from build123d import *

# Parameters (mm, degrees)
SKETCH2_R             = 25.4
BOSS_EXTRUDE2_DEPTH   = 6
SKETCH3_R             = 15
BOSS_EXTRUDE3_DEPTH   = 60.5
SKETCH4_R             = 10.315
CUT_EXTRUDE1_DEPTH    = 38.1
SKETCH5_R             = 7.07
CUT_EXTRUDE2_DEPTH    = 53.363441445
F_4_0MM_DOWEL_HOLE1_D = 4
CIRPATTERN1_COUNT     = 8
CIRPATTERN2_COUNT     = 6
CUT_EXTRUDE3_REACH    = 72.36


with BuildPart() as part:
    # Sketch2 → Boss-Extrude2 (new body)
    with BuildSketch(Plane(origin=(0, 0, 0), x_dir=(1, 0, 0), z_dir=(0, 1, 0))):
        with Locations(Location((0, 0, 0), (0, 0, 270))):
            Circle(SKETCH2_R)
    extrude(amount=BOSS_EXTRUDE2_DEPTH)

    # Sketch3 → Boss-Extrude3 (add)
    with BuildSketch(Plane.XZ):
        with Locations(Location((0, 0, 0), (0, 0, 270))):
            Circle(SKETCH3_R)
    extrude(amount=-BOSS_EXTRUDE3_DEPTH)

    # Sketch4 → Cut-Extrude1 (cut)
    with BuildSketch(Plane.XZ):
        with Locations(Location((0, 0, 0), (0, 0, 270))):
            Circle(SKETCH4_R)
    extrude(amount=-CUT_EXTRUDE1_DEPTH, mode=Mode.SUBTRACT)

    # Sketch5 → Cut-Extrude2 (cut, through all)
    with BuildSketch(Plane.XZ.offset(-38.1)):
        with Locations(Location((0, 0, 0), (0, 0, 270))):
            Circle(SKETCH5_R)
    extrude(amount=-CUT_EXTRUDE2_DEPTH, mode=Mode.SUBTRACT)

    # Ø4.0mm Dowel Hole1 (through all)
    with Locations(Plane(origin=(0, 0, 0), x_dir=(-1, 0, 0), z_dir=(0, -1, 0))):
        with Locations((0, 20.7)):
            f_4_0mm_dowel_hole1 = Hole(F_4_0MM_DOWEL_HOLE1_D / 2)

    # CirPattern1: Ø4.0mm Dowel Hole1 ×8 about axis
    cirpattern1_axis = Axis((0, 0, 0), (0, 1, 0))
    for i in range(1, CIRPATTERN1_COUNT):
        add(f_4_0mm_dowel_hole1.rotate(cirpattern1_axis, i * 360 / CIRPATTERN1_COUNT), mode=Mode.SUBTRACT)

    # Sketch13 → Ø3.0mm Dowel Hole1 (revolve, cut)
    with BuildSketch(Plane(origin=(-10.14, 60.5, 5.71), x_dir=(0, 0, 1), z_dir=(1, 0, 0))):
        Polygon((0, 0), (0, 6.201721238), (2, 5), (2, 0), align=None)
    f_3_0mm_dowel_hole1 = revolve(axis=Axis((-10.14, 66.85, 5.71), (0, -1, 0)), mode=Mode.SUBTRACT)

    # CirPattern2: Ø3.0mm Dowel Hole1 ×6 about axis
    cirpattern2_axis = Axis((0, 0, 0), (0, 1, 0))
    for i in range(1, CIRPATTERN2_COUNT):
        add(f_3_0mm_dowel_hole1.rotate(cirpattern2_axis, i * 360 / CIRPATTERN2_COUNT), mode=Mode.SUBTRACT)

    # Sketch14 → Cut-Extrude3 (cut, up to next)
    with BuildSketch(Plane(origin=(0, 60.5, 0), x_dir=(1, 0, 0), z_dir=(0, 1, 0)), mode=Mode.PRIVATE) as cut_extrude3_sk1:
        with BuildLine():
            Line((-2.5, 9.57), (2.5, 9.57))
            Line((2.5, 9.57), (2.5, 6.613236726))
            ThreePointArc((2.5, 6.613236726), (0, 7.07), (-2.5, 6.613236726))
            Line((-2.5, 6.613236726), (-2.5, 9.57))
        make_face()
    cut_extrude3_tool1 = extrude(cut_extrude3_sk1.sketch, amount=-CUT_EXTRUDE3_REACH, mode=Mode.PRIVATE) & part.part
    add(cut_extrude3_tool1.solids().sort_by_distance((0, 60.5, -8.24142))[0], mode=Mode.SUBTRACT)


solid = part.part
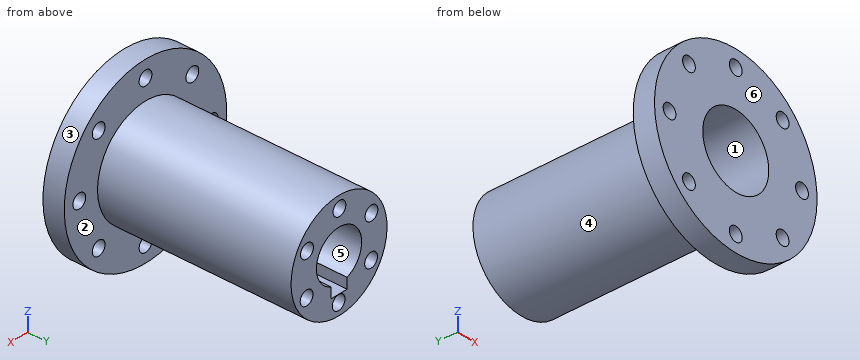
Check sheet for the modelled part. Datum: model origin and axes. Units: mm. Face numbers are marked on the shaded views. A direction names the side the tool comes from. Round coordinates to 2 decimals unless told otherwise and drop trailing zeros. Loops run counter-clockwise (first coordinate to the right, second up) from the corner with the lowest first, then second, coordinate; pieces in that order, holes last. Notation, with made-up numbers: M -27,54 L -15,54 A31 cw -15,91 Z; hole C 4,75.5 d9. An arc over 180 degrees is marked long. One line per item, written item: value.
(1) Sectioned sample at C-C, the plane x = -4. Record the cut outline in (y, z), then the cut area to 3 significant figures.
Computed values:
outline: M 0,-25.08 L 6,-25.08 L 6,-14.46 L 60.5,-14.46 L 60.5,-5.83 L 38.1,-5.83 L 38.1,-9.51 L 0,-9.51 Z; M 0,9.51 L 38.1,9.51 L 38.1,5.83 L 60.5,5.83 L 60.5,14.46 L 6,14.46 L 6,25.08 L 0,25.08 Z
area: 891 mm^2
(2) Depth check by flat-ended pin: pin 1 Ø1.5 at (x, y) = (11.5, 22.5) entering from -Z; pin 2 Ø10 at (y, z) = (22, -12) entering from +X; pin 3 Ø6.5 at (x, z) = (-14.64, -14.64) entering from +Y. Enter the tip coordinate at first touch or a pass-through.
Computed values:
pin 1: stops at z = -10.46
pin 2: stops at x = 13.27
pin 3: stops at y = 6
(3) Sectioned sample at D-D, the plane y = 8. Record the cut outline in (x, z) (3 decimals).
Computed values:
outline: C 0,0 d30; hole C 0,0 d20.63
(4) Access from +Z, -Z, +X, -X, +Y, -Y to the whole of each face (thin tool, end or side, straight path). Record for the marked faces 1, 2 and 3.
Computed values:
face 1: -Y
face 2: +Y
face 3: +Y, -Y
(5) Sectioned sample at B-B, the plane z = -20.7. Record the cut outline in (x, y), then the cut area to 3 significant figures.
Computed values:
outline: M -14.72,0 L -2,0 L -2,6 L -14.72,6 Z; M 2,0 L 14.72,0 L 14.72,6 L 2,6 Z
area: 153 mm^2
(6) Sectioned sample at A-A, the plane y = 53. Record the cut outline in (x, z), then the cut area to 3 significant figures.
Computed values:
outline: C 0,0 d30; hole M -2.5,-9.57 L 2.5,-9.57 L 2.5,-6.61 A7.07 ccw long -2.5,-6.61 Z
area: 537 mm^2
(7) Thickness scan on line 1 (X direction, y = 2, z = 0) (3 decimals); line 2 (X direction, y = 12, z = 0) (3 decimals); line 3 (Y direction, x = 21.5, z = -13). Record the ranges inside material, lowest first.
Computed values:
line 1: x = -25.4 to -22.7, -18.7 to -10.315, 10.315 to 18.7, 22.7 to 25.4
line 2: x = -15 to -10.315, 10.315 to 15
line 3: y = 0 to 6
(8) Release check for a two-part mould opening along X. For the marked faces 4, 5 and 6 record: +X half, -X half, draft (parallel to the pull), parting line (faces both ways), or undercut.
Computed values:
face 4: parting line
face 5: undercut
face 6: draft
